Input: dimensioned drawing with shaded views. Units: mm. Origin: part minimum x, y, z. A direction names the side the tool comes from. Give positions to 0.01 mm unless a question says otherwise; leave off trailing zeros. Order: outer loops, then holes, each group sorted by start corner. A loop starts at its lowest first (then second) coordinate and runs counter-clockwise, first axis right, second up. Notation, with made-up numbers: (-14.75, 55.25) - (7.25, 55.25) arc R26 ccw to (7.25, 90.25) - close; hole circle Ø11 at (-36.75, -38.5). An arc over 180 degrees is marked (long way). Use a Markdown table: item, result.
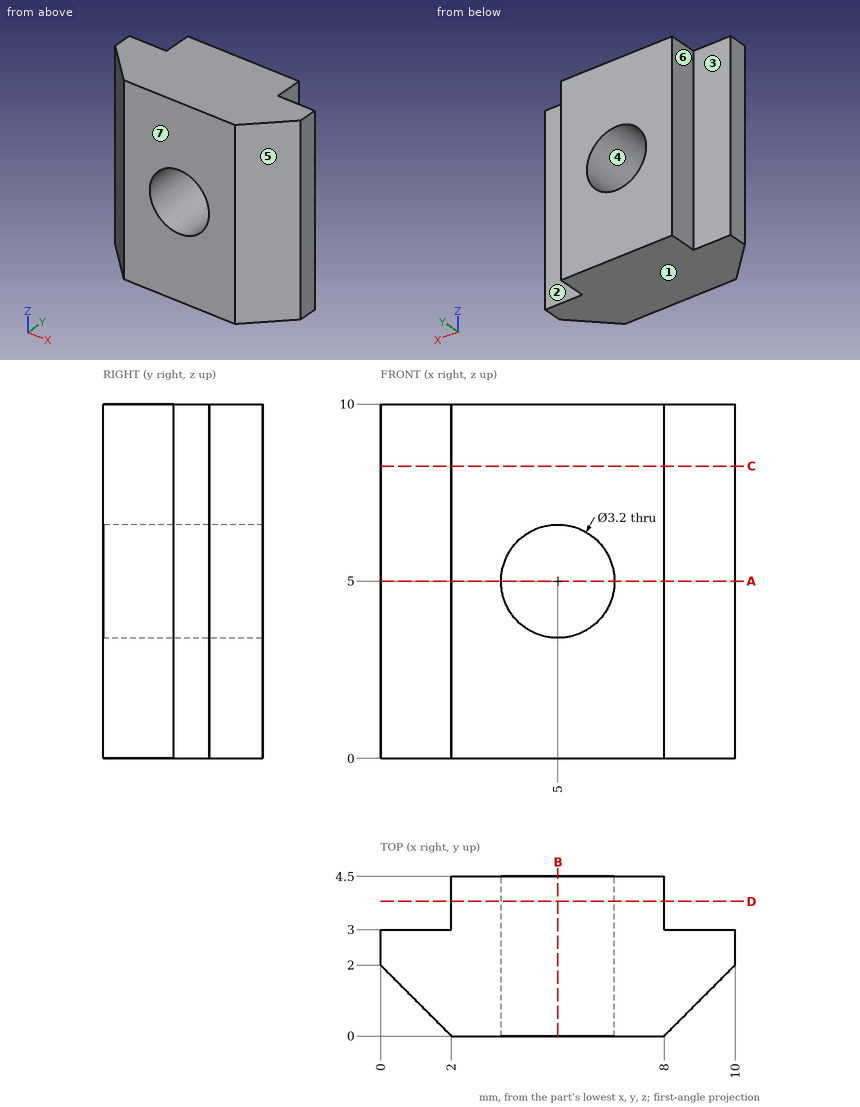
1. Material intervals for line 1 along X through (y, z) = (2.7, 5); line 2 along X through (y, z) = (4.2, 0.5); line 3 along Z through (x, y) = (4.75, 2.2), sorted ascending.
Response:
| item | result |
|---|---|
| line 1 | x = 0 to 3.4, 6.6 to 10 |
| line 2 | x = 2 to 8 |
| line 3 | z = 0 to 3.42, 6.58 to 10 |
2. Section query D-D (y = 3.8). Return loops of the section in (x, z).
Response:
| item | result |
|---|---|
| outline | (2, 0) - (8, 0) - (8, 10) - (2, 10) - close; hole circle Ø3.2 at (5, 5) |
3. Section query B-B (x = 5). Return loops of the section in (y, z).
Response:
| item | result |
|---|---|
| outline | (0, 0) - (4.5, 0) - (4.5, 3.4) - (0, 3.4) - close; (0, 6.6) - (4.5, 6.6) - (4.5, 10) - (0, 10) - close |
4. Set-up query: the marked faces 1, 2 and 3. Return all of +Z, -Z, +X, -X, +Y, -Y with unobstructed straight access to the full face (end or side cutting, diameter ignored); none if empty.
Response:
| item | result |
|---|---|
| face 1 | -Z, +X, -X, +Y, -Y |
| face 2 | +Z, -Z, +X, +Y |
| face 3 | +Z, -Z, -X, +Y |
5. Section query A-A (z = 5). Return loops of the section in (x, y), then the cut area to 3 significant figures.
Response:
| item | result |
|---|---|
| outline | (0, 2) - (2, 0) - (3.4, 0) - (3.4, 4.5) - (2, 4.5) - (2, 3) - (0, 3) - close; (6.6, 0) - (8, 0) - (10, 2) - (10, 3) - (8, 3) - (8, 4.5) - (6.6, 4.5) - close |
| area | 20.6 mm^2 |
6. Section query C-C (z = 8.25). Return loops of the section in (x, y), then the cut area to 3 significant figures.
Response:
| item | result |
|---|---|
| outline | (0, 2) - (2, 0) - (8, 0) - (10, 2) - (10, 3) - (8, 3) - (8, 4.5) - (2, 4.5) - (2, 3) - (0, 3) - close |
| area | 35.0 mm^2 |
7. Mould query, pull axis X, two halves, no side actions, for the marked faces 4, 5, 6 and 7. Classes: pulls with the +X half, pulls with the -X half, needs draft (parallel to the pull), parting line crosses it, or undercut.
Response:
| item | result |
|---|---|
| face 4 | undercut |
| face 5 | pulls with the +X half |
| face 6 | pulls with the -X half |
| face 7 | needs draft |
8. Pin query (flat end, axial travel): pin 1 (1 mm diameter, centred on x = 0.5, z = 5.5, fed in from +Y); pin 2 (1.5 mm diameter, centred on y = 1, z = 7, fed in from +X); pin 3 (1.2 mm diameter, centred on y = 4, z = 6, fed in from -X). Return the tip coordinate at first contact, or that it passes through.
Response:
| item | result |
|---|---|
| pin 1 | stops at y = 3 |
| pin 2 | stops at x = 9.75 |
| pin 3 | stops at x = 2 |
